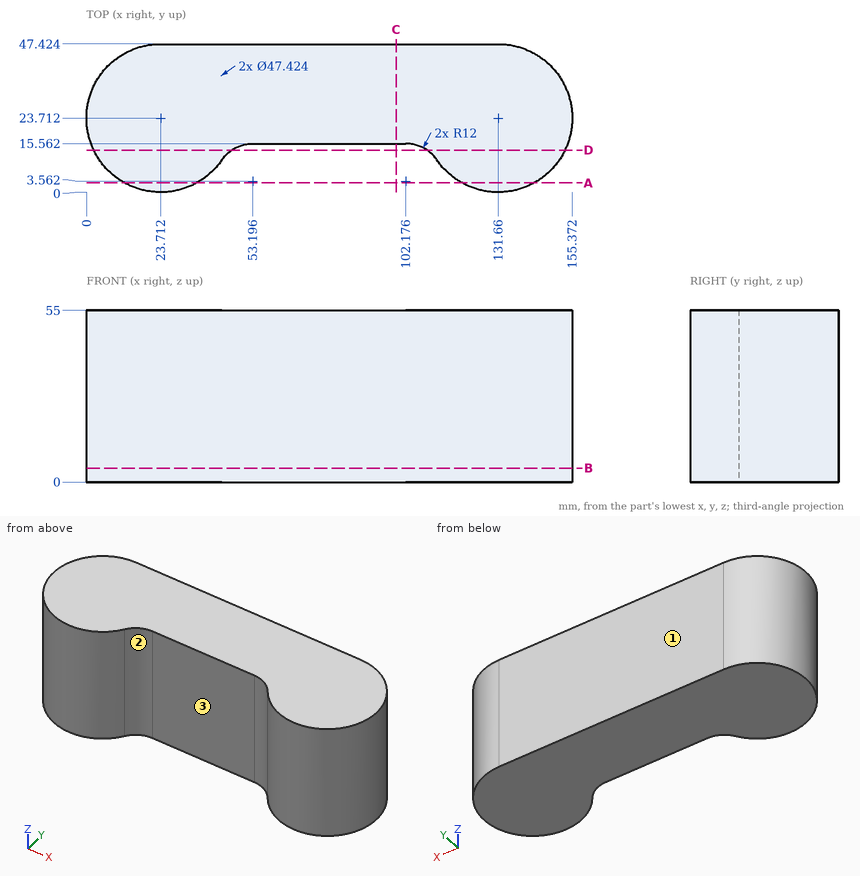
Source: three-view drawing plus pictorial views. Frame: mm from the lowest corner of the part. Round coordinates to 2 decimals unless told otherwise and drop trailing zeros. Order: outer loops, then holes, each group sorted by start corner. A loop starts at its lowest first (then second) coordinate and runs counter-clockwise, first axis right, second up. Notation, with made-up numbers: (34.5, 51.5) -> (71.5, 51.5) arc R20 ccw to (71.5, 72.5) -> close; hole circle Ø11 at (87, 49). An arc over 180 degrees is marked (long way). Use one line per item in the form item = value. Start each with the question number.
1. Cut plane C-C (x = 99). Return the cut outline in (y, z), then the cut area to 3 significant figures.
2. Line query: probe 1 along Y at (x, z) = (61.5, 40.5); probe 2 along X at (y, z) = (14, 7.5) (1 decimal); probe 3 along X at (y, z) = (24, 34). Output: solid intervals per line, ascending.
3. Pin query (flat end, axial travel): pin 1 Ø12 at (y, z) = (31.5, 10.5) entering from -X; pin 2 Ø1 at (x, z) = (21, 9) entering from +Y; pin 3 Ø14.5 at (x, z) = (83.5, 24) entering from -Y. Return the tip coordinate at first contact, or that it passes through.
4. Cut plane B-B (z = 4.5). Return the cut outline in (x, y), then the cut area to 3 significant figures.
5. Draft query along X for the marked faces 1, 2 and 3. Return one class per face: pulls with the +X half, pulls with the -X half, needs draft (parallel to the pull), parting line crosses it, or undercut.
6. Cut plane D-D (y = 13.5). Return the cut outline in (x, z).
7. Cut plane A-A (y = 3). Return the cut outline in (x, z) (1 decimal), then the cut area to 3 significant figures.
Solution:
q1.outline = (15.56, 0) -> (47.42, 0) -> (47.42, 55) -> (15.56, 55) -> close
q1.area = 1,750 mm^2
q2.probe_1 = 15.56 to 47.42
q2.probe_2 = 2.1 to 47.3, 108.1 to 153.3
q2.probe_3 = 0 to 155.37
q3.pin_1 = 0.07
q3.pin_2 = 47.32
q3.pin_3 = 15.56
q4.outline = (23.71, 47.42) arc R23.71 ccw (long way) to (43.29, 10.33) arc R12 cw to (53.2, 15.56) -> (102.18, 15.56) arc R12 cw to (112.08, 10.33) arc R23.71 ccw (long way) to (131.66, 47.42) -> close
q4.area = 5,730 mm^2
q5.face_1 = needs draft
q5.face_2 = undercut
q5.face_3 = undercut
q6.outline = (2.31, 0) -> (46.47, 0) -> (46.47, 55) -> (2.31, 55) -> close; (108.9, 0) -> (153.06, 0) -> (153.06, 55) -> (108.9, 55) -> close
q7.outline = (12.2, 0) -> (35.3, 0) -> (35.3, 55) -> (12.2, 55) -> close; (120.1, 0) -> (143.2, 0) -> (143.2, 55) -> (120.1, 55) -> close
q7.area = 2,540 mm^2
